```python
from build123d import *

# Parameters (mm, degrees)
SKETCH1_W                                           = 50.8
SKETCH1_H                                           = 25.4
BOSS_EXTRUDE1_DEPTH                                 = 26.9875
CBORE_FOR_0_BINDING_HEAD_MACHINE_SCREW1_D           = 6.35
CBORE_FOR_0_BINDING_HEAD_MACHINE_SCREW1_CBORE_D     = 15.875
CBORE_FOR_0_BINDING_HEAD_MACHINE_SCREW1_CBORE_DEPTH = 9.525


with BuildPart() as part:
    # Sketch1 → Boss-Extrude1 (new body)
    with BuildSketch(Plane.XY):
        Rectangle(SKETCH1_W, SKETCH1_H)
    extrude(amount=-BOSS_EXTRUDE1_DEPTH)

    # CBORE for #0 Binding Head Machine Screw1 (through all)
    with Locations(Plane(origin=(0, 0, -26.9875), x_dir=(-1, 0, 0), z_dir=(0, 0, -1))):
        with Locations((0, 0)):
            CounterBoreHole(CBORE_FOR_0_BINDING_HEAD_MACHINE_SCREW1_D / 2, CBORE_FOR_0_BINDING_HEAD_MACHINE_SCREW1_CBORE_D / 2, CBORE_FOR_0_BINDING_HEAD_MACHINE_SCREW1_CBORE_DEPTH)


solid = part.part
```
For this review, take the finished solid that the model builds, in its own axes (mm). A direction names the side the tool comes from. Round coordinates to 2 decimals unless told otherwise and drop trailing zeros. Write each loop counter-clockwise with the first axis right and the second up, starting at its lowest first coordinate (ties: lowest second). Pieces come first, ordered by that corner, then holes. Notation, with made-up numbers: (63, 4) -> (82, 4) arc R18 cw to (82, 35) -> close; hole circle Ø9 at (32.25, 54). An arc over 180 degrees is marked (long way). One line per question, with ' | ' between items. Start each with the question number.
(1) Mouldability with a two-part tool opening along X and no side actions: class faces 1 (the face through (0, -12.7, -13)), 2 (the face through (1.72, -7.75, -22.29)), 3 (the face through (25.4, 0, -13)) as released by +X, released by -X, zero draft, split by the parting line, or undercut.
(2) Add section A-A, the plane x = 0. Write out the cut boundary in (y, z) (1 decimal), plus the area to 3 significant figures.
(3) Add section B-B, the plane y = 0. Write out the cut boundary in (x, z) (1 decimal).
(4) Add section D-D, the plane z = -24.5. Write out the cut boundary in (x, y) (1 decimal).
(5) Add section C-C, the plane z = -8.75. Write out the cut boundary in (x, y) (3 decimals), plus the area to 3 significant figures.
(6) Tool access review of faces 4 (the face through (-3.4, 0.1, -17.462)), 5 (the face through (-25.4, 0, -13)): name each direction out of +Z, -Z, +X, -X, +Y, -Y from which nothing blocks a thin tool from reaching the whole face with its end or side.
(7) Insertion check: P1, Ø5.5, axis at x = 0, y = 0, coming from the +Z side. The pin has a flat end and moves straight along its axis. Give the tip position at first contact, or say it passes through.
(8) For line 1 along X through (y, z) = (-0.25, -16.25); line 2 along Y through (x, z) = (0, -9.5) (3 decimals); line 3 along X through (y, z) = (-3, -24.5), list the stretches that pass through material, from the lowest coordinate up. Write a range as from..to.
Answer list:
1) face 1: zero draft | face 2: undercut | face 3: released by +X
2) outline: (-12.7, -27) -> (-7.9, -27) -> (-7.9, -17.5) -> (-3.2, -17.5) -> (-3.2, 0) -> (-12.7, 0) -> close; (3.2, -17.5) -> (7.9, -17.5) -> (7.9, -27) -> (12.7, -27) -> (12.7, 0) -> (3.2, 0) -> close | area: 423 mm²
3) outline: (-25.4, -27) -> (-7.9, -27) -> (-7.9, -17.5) -> (-3.2, -17.5) -> (-3.2, 0) -> (-25.4, 0) -> close; (3.2, -17.5) -> (7.9, -17.5) -> (7.9, -27) -> (25.4, -27) -> (25.4, 0) -> (3.2, 0) -> close
4) outline: (-25.4, -12.7) -> (25.4, -12.7) -> (25.4, 12.7) -> (-25.4, 12.7) -> close; hole circle Ø15.9 at (0, 0)
5) outline: (-25.4, -12.7) -> (25.4, -12.7) -> (25.4, 12.7) -> (-25.4, 12.7) -> close; hole circle Ø6.35 at (0, 0) | area: 1,260 mm²
6) face 4: -Z | face 5: +Z, -Z, -X, +Y, -Y
7) P1: through
8) line 1: -25.4..-3.17, 3.17..25.4 | line 2: -12.7..-3.175, 3.175..12.7 | line 3: -25.4..-7.35, 7.35..25.4
